Could you check a few things on this model? Use its own coordinates, in mm. Give positions to 0.01 mm unless a question says otherwise; leave off trailing zeros. Loops run counter-clockwise (first coordinate to the right, second up) from the corner with the lowest first, then second, coordinate; pieces in that order, holes last. Notation, with made-up numbers: M 62,40.5 L 120,40.5 A28 cw 120,67.5 Z; hole C 25.5,55 d11. An arc over 180 degrees is marked long. Use a Markdown table: item, result. Add a question column.
1) Suppose I cut it at C-C on y = -46. List the corners of the cut face in (x, z) for me.
2) Suppose I cut it at B-B on z = 0.45. Count the separate pieces of the cut face and the enclosed holes in it, and give its area (3 significant figures).
3) Suppose I cut it at A-A on y = 19.5. List the corners of the cut face in (x, z) for me, and give its area (4 significant figures).
4) Will these pins go through, and if not, where does the flat tip stop? pin 1 Ø0.8 at (x, z) = (40.5, 1) entering from -Y; pin 2 Ø1 at (x, z) = (-45, 1.5) entering from +Y; pin 3 Ø1.2 at (x, z) = (-47.5, 1) entering from -Y.
5) If I drill on line 1 along X through (y, z) = (19, 0.7); line 2 along Y through (x, z) = (28.75, 1.95); line 3 along Y through (x, z) = (37, 0.6), over which ranges is the centre line in solid material (lowest first)? Write a range as [from, to].
```python
from build123d import *

# Parameters (mm, degrees)
RESSALTO_EXTRUS_O1_DEPTH = 2.5
ESBO_O2_R                = 1.15
CORTE_EXTRUS_O1_DEPTH    = 90.837353033
ESBO_O4_R                = 1.65
CORTE_EXTRUS_O2_DEPTH    = 40.5


with BuildPart() as part:
    # Esboço1 → Ressalto-extrusão1 (new body)
    with BuildSketch(Plane.XY):
        Polygon((63.5, -26.302561211), (63.5, 26.302561211), (26.302561211, 63.5), (-26.302561211, 63.5), (-63.5, 26.302561211), (-63.5, -26.302561211), (-26.302561211, -63.5), (26.302561211, -63.5), align=None)
    extrude(amount=RESSALTO_EXTRUS_O1_DEPTH)

    # Esboço2 → Corte-extrusão1 (cut, through all)
    with BuildSketch(Plane(origin=(0, 0, 0), x_dir=(-1, 0, 0), z_dir=(0, 0, -1))):
        with Locations((28.75, 8.5)):
            Circle(ESBO_O2_R)
        with Locations(Location((28.75, -8.5, 0), (0, 0, 180))):
            Circle(ESBO_O2_R)
        with Locations((-28.75, -8.5)):
            Circle(ESBO_O2_R)
        with Locations(Location((-28.75, 8.5, 0), (0, 0, 180))):
            Circle(ESBO_O2_R)
        with Locations((-6.731, -57)):
            Circle(ESBO_O2_R)
        with Locations(Location((6.731, -57, 0), (0, 0, 180))):
            Circle(ESBO_O2_R)
        with Locations((6.731, 57)):
            Circle(ESBO_O2_R)
        with Locations(Location((-6.731, 57, 0), (0, 0, 180))):
            Circle(ESBO_O2_R)
        with BuildLine():
            Line((54, 24), (36, 24))
            ThreePointArc((36, 24), (33.878679656, 23.121320344), (33, 21))
            Line((33, 21), (33, -21))
            ThreePointArc((33, -21), (33.878679656, -23.121320344), (36, -24))
            Line((36, -24), (54, -24))
            ThreePointArc((54, -24), (56.121320344, -23.121320344), (57, -21))
            Line((57, -21), (57, 21))
            ThreePointArc((57, 21), (56.121320344, 23.121320344), (54, 24))
        make_face()
        with BuildLine():
            Line((-33, 21), (-33, -21))
            ThreePointArc((-33, -21), (-33.878679656, -23.121320344), (-36, -24))
            Line((-36, -24), (-54, -24))
            ThreePointArc((-54, -24), (-56.121320344, -23.121320344), (-57, -21))
            Line((-57, -21), (-57, 21))
            ThreePointArc((-57, 21), (-56.121320344, 23.121320344), (-54, 24))
            Line((-54, 24), (-36, 24))
            ThreePointArc((-36, 24), (-33.878679656, 23.121320344), (-33, 21))
        make_face()
    extrude(amount=-CORTE_EXTRUS_O1_DEPTH, mode=Mode.SUBTRACT)

    # Esboço4 → Corte-extrusão2 (cut)
    with BuildSketch(Plane(origin=(0, 0, 0), x_dir=(-1, 0, 0), z_dir=(0, 0, -1))):
        with Locations((36.062445841, -36.062445841)):
            Circle(ESBO_O4_R)
        with Locations((36.062445841, 36.062445841)):
            Circle(ESBO_O4_R)
        with Locations((-36.062445841, -36.062445841)):
            Circle(ESBO_O4_R)
        with Locations((-36.062445841, 36.062445841)):
            Circle(ESBO_O4_R)
    extrude(amount=-CORTE_EXTRUS_O2_DEPTH, mode=Mode.SUBTRACT)


solid = part.part
```
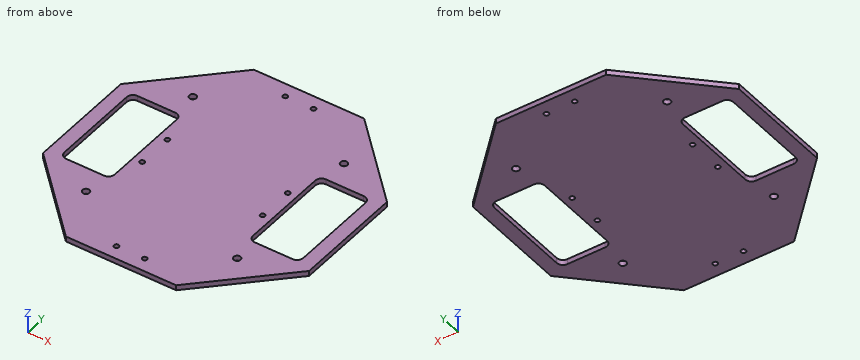
Answer block:
| question | item | result |
|---|---|---|
| 1 | outline | M -43.8,0 L 43.8,0 L 43.8,2.5 L -43.8,2.5 Z |
| 2 | separate pieces | 1 |
| 2 | enclosed holes | 14 |
| 2 | area | 11,000 mm^2 |
| 3 | outline | M -63.5,0 L -57,0 L -57,2.5 L -63.5,2.5 Z; M -33,0 L 33,0 L 33,2.5 L -33,2.5 Z; M 57,0 L 63.5,0 L 63.5,2.5 L 57,2.5 Z |
| 3 | area | 197.5 mm^2 |
| 4 | pin 1 | stops at y = -49.7 |
| 4 | pin 2 | stops at y = 45.3 |
| 4 | pin 3 | stops at y = -42.9 |
| 5 | line 1 | x = [-63.5, -57], [-33, 33], [57, 63.5] |
| 5 | line 2 | y = [-61.05, -9.65], [-7.35, 7.35], [9.65, 61.05] |
| 5 | line 3 | y = [-52.8, -37.42], [-34.7, -24], [24, 34.7], [37.42, 52.8] |
